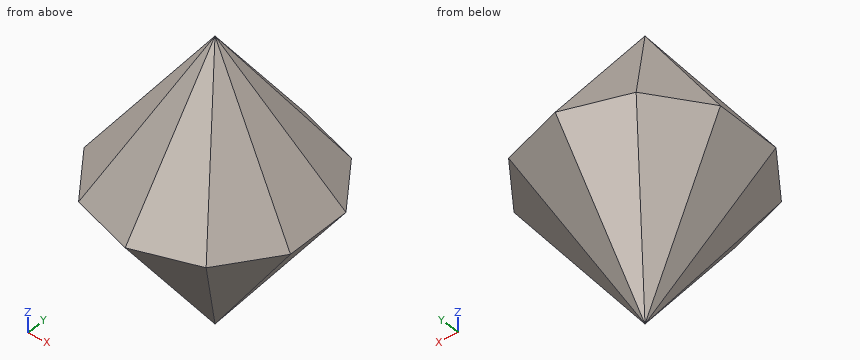
from build123d import *

# Parameters (mm, degrees)
F1_DEPTH  = 30
F7_DEPTH  = 67.083039
F8_DEPTH  = 67.083039
F9_DEPTH  = 62.189471
F10_DEPTH = 58.648451
F11_DEPTH = 61.353549


with BuildPart() as f1:
    # F0 (on Top) → F1 (new body, symmetric)
    with BuildSketch(Plane.XY):
        Polygon((21.796276, 30), (-21.796276, 30), (-35.267115, -11.45898), (0, -37.082039), (35.267115, -11.45898), align=None)
    extrude(amount=F1_DEPTH, both=True)

    # F2 (on face) → F7 (intersect, through all)
    with BuildSketch(Plane(origin=(0, 30, 0), x_dir=(-1, 0, 0), z_dir=(0, 1, 0))):
        Polygon((21.796276, 0), (0, 30), (-21.796276, 0), (0, -30), align=None)
    extrude(amount=-F7_DEPTH, mode=Mode.INTERSECT)

    # F3 (on face) → F8 (intersect, through all)
    with BuildSketch(Plane(origin=(-17.633558, -24.27051, 0), x_dir=(0.809017, -0.587785, 0), z_dir=(-0.587785, -0.809017, 0))):
        Polygon((0, 30), (-21.796276, 0), (0, -30), (21.796276, 0), align=None)
    extrude(amount=-F8_DEPTH, mode=Mode.INTERSECT)

    # F4 (on face) → F9 (intersect, through all)
    with BuildSketch(Plane(origin=(-28.531695, 9.27051, 0), x_dir=(-0.309017, -0.951057, 0), z_dir=(-0.951057, 0.309017, 0))):
        Polygon((0, -30), (21.796276, 0), (0, 30), (-21.796276, 0), align=None)
    extrude(amount=-F9_DEPTH, mode=Mode.INTERSECT)

    # F5 (on face) → F10 (intersect, through all)
    with BuildSketch(Plane(origin=(28.531695, 9.27051, 0), x_dir=(-0.309017, 0.951057, 0), z_dir=(0.951057, 0.309017, 0))):
        Polygon((0, -30), (21.796276, 0), (0, 30), (-21.796276, 0), align=None)
    extrude(amount=-F10_DEPTH, mode=Mode.INTERSECT)

    # F6 (on face) → F11 (intersect, through all)
    with BuildSketch(Plane(origin=(17.633558, -24.27051, 0), x_dir=(0.809017, 0.587785, 0), z_dir=(0.587785, -0.809017, 0))):
        Polygon((0, -30), (21.796276, 0), (0, 30), (-21.796276, 0), align=None)
    extrude(amount=-F11_DEPTH, mode=Mode.INTERSECT)


solid = f1.part
Can you work these out from the model? Positions are in its coordinate system, mm. Round coordinates to 2 decimals unless told otherwise and drop trailing zeros. Order: outer loops, then holes, each group sorted by start corner. A loop starts at its lowest first (then second) coordinate and runs counter-clockwise, first axis right, second up. Notation, with made-up numbers: (2, 62.5) - (44, 62.5) arc R19 ccw to (44, 76.5) - close; hole circle Ø4 at (64.25, -37). An arc over 180 degrees is marked (long way). Answer in a Markdown table with one row per item.
(1) Suppose I cut it at B-B, the plane z = 15. Please give me the cut outline in (x, y).
From the geometry:
| item | result |
|---|---|
| outline | (-10.9, -3.54) - (-6.74, -9.27) - (0, -11.46) - (6.74, -9.27) - (10.9, -3.54) - (10.9, 3.54) - (6.74, 9.27) - (0, 11.46) - (-6.74, 9.27) - (-10.9, 3.54) - close |
(2) Please list where these lines run through material, in increasing order: L1, parallel to X at y = 5, z = -0.5; L2, parallel to Z at x = 8, y = -19; L3, parallel to Y at x = -17.5, z = 2.5. Write a range as from..to.
From the geometry:
| item | result |
|---|---|
| L1 | x = -21.43..21.43 |
| L2 | z = -1.73..1.73 |
| L3 | y = -9.91..9.91 |
(3) Suppose I cut it at A-A, the plane y = -9. Please give me the cut outline in (x, z), plus the area to 3 significant figures.
From the geometry:
| item | result |
|---|---|
| outline | (-20.4, 0) - (-6.54, -15.44) - (0, -18.22) - (6.54, -15.44) - (20.4, 0) - (6.54, 15.44) - (0, 18.22) - (-6.54, 15.44) - close |
| area | 868 mm2 |
(4) Suppose I cut it at C-C, the plane x = -6. Please give me the cut outline in (y, z), plus the area to 3 significant figures.
From the geometry:
| item | result |
|---|---|
| outline | (-20.97, 0) - (-8.26, -16.64) - (-1.95, -21.74) - (1.95, -21.74) - (8.26, -16.64) - (20.97, 0) - (8.26, 16.64) - (1.95, 21.74) - (-1.95, 21.74) - (-8.26, 16.64) - close |
| area | 1,080 mm2 |
(5) For P1, Ø8, axis at x = -1.5, y = 14, coming from the -Z side; P2, Ø6, axis at x = 5, z = -5, coming from the -Y side; P3, Ø5, axis at x = 16.5, y = -18, coming from the +Z side; P4, Ø2, axis at x = -11, z = -18, coming from the +Y side, each with a flat end and sliding along its axis, tell me the tip position at first contact or that it passes through.
From the geometry:
| item | result |
|---|---|
| P1 | stops at z = -16.54 |
| P2 | stops at y = -19.96 |
| P3 | stops at z = 0.51 |
| P4 | passes through |
(6) Suppose I cut it at D-D, the plane y = 13. Please give me the cut outline in (x, z).
From the geometry:
| item | result |
|---|---|
| outline | (-17.5, 0) - (-9.45, -8.97) - (0, -12.98) - (9.45, -8.97) - (17.5, 0) - (9.45, 8.97) - (0, 12.98) - (-9.45, 8.97) - close |
